The listing builds one solid part. Answer for the finished solid, in the listing's coordinates (mm). Coordinates: 2 decimals unless noted, no trailing zeros. Loops run counter-clockwise (first coordinate to the right, second up) from the corner with the lowest first, then second, coordinate; pieces in that order, holes last. Notation, with made-up numbers: M 5.5,13 L 43.5,13 A27 cw 43.5,50 Z; hole C 46,11.25 d1. An arc over 180 degrees is marked long. Return JSON: item names as keys, results as strings. Group by question number.
1. Section C-C (x = -6.75) is taken. Write down the section's boundary in (y, z) (3 decimals).
2. Section D-D (z = 18.25) is taken. Write down the section's boundary in (x, y) (3 decimals), then the cut area to 3 significant figures.
3. The mould has two halves that part along Y. Classify faces 1 (the face through (-5, 2, 0)), 2 (the face through (-3.446, 3.16, 3.88)), 3 (the face through (0, -10.16, 10)): pulls with the +Y half, pulls with the -Y half, needs draft (parallel to the pull), parting line crosses it, or undercut.
4. Straight lines are drawn through the part: L1, parallel to Y at x = 5.5, z = 10.16 (3 decimals); L2, parallel to X at y = 0.5, z = 3.25. For each, find the intervals that lie inside material, in ascending order. Write a range as from..to.
5. Section A-A (y = 0) is taken. Write down the section's boundary in (x, z) (3 decimals), then the cut area to 3 significant figures.
6. Section B-B (z = 12) is taken. Write down the section's boundary in (x, y) (3 decimals).
```python
from build123d import *

# Parameters (mm, degrees)
SKETCH1_W                      = 20.32
SKETCH1_H                      = 20.32
SKETCH1_R                      = 4.675
BOSS_EXTRUDE1_DEPTH            = 20.32
F_20_0_20_DIAMETER_HOLE1_D     = 9.35
F_20_0_20_DIAMETER_HOLE1_DEPTH = 20.32
F_20_0_20_DIAMETER_HOLE1_TIP   = 2.809023394


with BuildPart() as part:
    # Sketch1 → Boss-Extrude1 (new body)
    with BuildSketch(Plane.XY):
        Rectangle(SKETCH1_W, SKETCH1_H)
        Circle(SKETCH1_R, mode=Mode.SUBTRACT)
    extrude(amount=BOSS_EXTRUDE1_DEPTH)

    # Ø20.0 (20) Diameter Hole1
    with Locations(Plane(origin=(10.16, 0, 0), x_dir=(0, 0, -1), z_dir=(1, 0, 0))):
        with Locations((-10.16, 0)):
            Hole(F_20_0_20_DIAMETER_HOLE1_D / 2, depth=F_20_0_20_DIAMETER_HOLE1_DEPTH)
            with Locations((0, 0, -(F_20_0_20_DIAMETER_HOLE1_DEPTH + F_20_0_20_DIAMETER_HOLE1_TIP / 2))):  # 118° drill point
                Cone(0, F_20_0_20_DIAMETER_HOLE1_D / 2, F_20_0_20_DIAMETER_HOLE1_TIP, mode=Mode.SUBTRACT)


solid = part.part
```
Worked out:
{
 "1": {"outline": "M -10.16,0 L 10.16,0 L 10.16,20.32 L -10.16,20.32 Z; hole C 0,10.16 d9.35"},
 "2": {"outline": "M -10.16,-10.16 L 10.16,-10.16 L 10.16,10.16 L -10.16,10.16 Z; hole C 0,0 d9.35", "area": "344 mm^2"},
 "3": {"face 1": "needs draft", "face 2": "undercut", "face 3": "pulls with the -Y half"},
 "4": {"L1": "-10.16..-4.675, 4.675..10.16", "L2": "-10.16..-4.65, 4.65..10.16"},
 "5": {"outline": "M -10.16,0 L -4.675,0 L -4.675,5.485 L -10.16,5.485 Z; M -10.16,14.835 L -4.675,14.835 L -4.675,20.32 L -10.16,20.32 Z; M 4.675,0 L 10.16,0 L 10.16,5.485 L 4.675,5.485 Z; M 4.675,14.835 L 10.16,14.835 L 10.16,20.32 L 4.675,20.32 Z", "area": "120 mm^2"},
 "6": {"outline": "M -10.16,-10.16 L 10.16,-10.16 L 10.16,-4.298 L 1.84,-4.298 A4.675 cw -1.84,-4.298 L -10.16,-4.298 Z; M -10.16,4.298 L -1.84,4.298 A4.675 cw 1.84,4.298 L 10.16,4.298 L 10.16,10.16 L -10.16,10.16 Z"}
}
